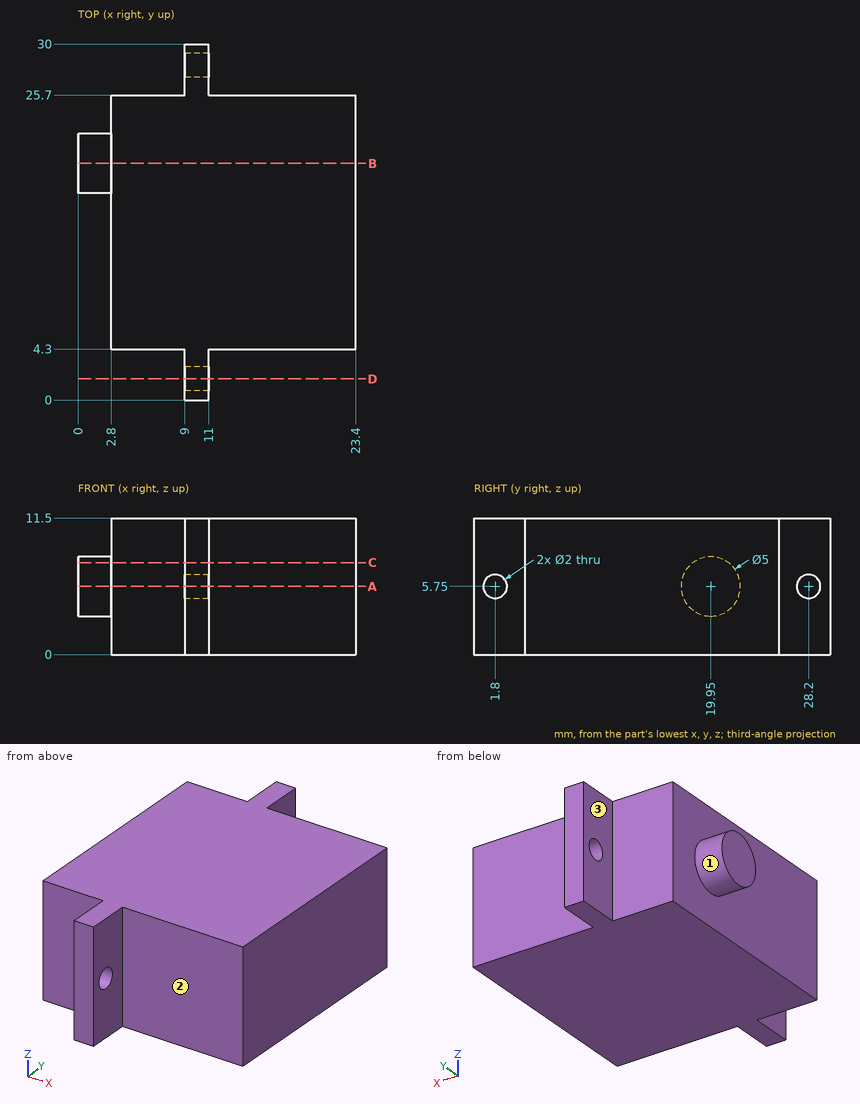
Design review of the part shown in the three views and the two pictorial views. Dimensions are in mm from the part's minimum x, y and z. A direction names the side the tool comes from. Give positions to 0.01 mm unless a question says otherwise; leave off trailing zeros. Loops run counter-clockwise (first coordinate to the right, second up) from the corner with the lowest first, then second, coordinate; pieces in that order, holes last. Notation, with made-up numbers: M 55.25,14 L 108.25,14 A28 cw 108.25,40 Z; hole C 81,21 d3. An arc over 180 degrees is marked long. Write item = value, one per line.
Q1. We need section C-C (z = 7.75). Give the boundary of the cut face in (x, y), plus the area to 3 significant figures.
Output values:
outline = M 0,18.45 L 2.8,18.45 L 2.8,4.3 L 9,4.3 L 9,0 L 11,0 L 11,4.3 L 23.4,4.3 L 23.4,25.7 L 11,25.7 L 11,30 L 9,30 L 9,25.7 L 2.8,25.7 L 2.8,21.45 L 0,21.45 Z
area = 466 mm^2
Q2. For the marked faces 1, 2 and 3, list the 3-axis set-ups (+Z, -Z, +X, -X, +Y, -Y) from which the entire face can be reached by the end or side of a thin tool; tool diameter is ignored.
Output values:
face_1 = -X
face_2 = +Z, -Z, +X, -Y
face_3 = +Z, -Z, -X, +Y
Q3. We need section B-B (y = 19.95). Give the boundary of the cut face in (x, z), plus the area to 3 significant figures.
Output values:
outline = M 0,3.25 L 2.8,3.25 L 2.8,0 L 23.4,0 L 23.4,11.5 L 2.8,11.5 L 2.8,8.25 L 0,8.25 Z
area = 251 mm^2
Q4. We need section D-D (y = 1.8). Give the boundary of the cut face in (x, z).
Output values:
outline = M 9,0 L 11,0 L 11,4.75 L 9,4.75 Z; M 9,6.75 L 11,6.75 L 11,11.5 L 9,11.5 Z
Q5. Insertion check: pin 1 (5 mm diameter, centred on x = 6, z = 3.5, fed in from -Y); pin 2 (1.3 mm diameter, centred on y = 3, z = 5.5, fed in from -X); pin 3 (2 mm diameter, centred on y = 26.5, z = 4.5, fed in from -X). Each pin has a flat end and moves straight along its axis. Give the tip position at first contact, or say it passes through.
Output values:
pin_1 = 4.3
pin_2 = 9
pin_3 = 2.8
Q6. To check wall thickness, follow line 1 (Y direction, x = 9.45, z = 5.75); line 2 (X direction, y = 7, z = 11.25); line 3 (Y direction, x = 13.25, z = 10.25). State the ranges of each line that lie inside material, in increasing order. Write a range as [from, to].
Output values:
line_1 = [0, 0.8], [2.8, 27.2], [29.2, 30]
line_2 = [2.8, 23.4]
line_3 = [4.3, 25.7]
Q7. We need section A-A (z = 5.75). Give the boundary of the cut face in (x, y).
Output values:
outline = M 0,17.45 L 2.8,17.45 L 2.8,4.3 L 9,4.3 L 9,2.8 L 11,2.8 L 11,4.3 L 23.4,4.3 L 23.4,25.7 L 11,25.7 L 11,27.2 L 9,27.2 L 9,25.7 L 2.8,25.7 L 2.8,22.45 L 0,22.45 Z; M 9,0 L 11,0 L 11,0.8 L 9,0.8 Z; M 9,29.2 L 11,29.2 L 11,30 L 9,30 Z
